Could you check a few things on this drawing? It's one solid part, dimensions in mm from its lowest x, y, z. A direction names the side the tool comes from. Round coordinates to 2 decimals unless told otherwise and drop trailing zeros. Loops run counter-clockwise (first coordinate to the right, second up) from the corner with the lowest first, then second, coordinate; pieces in that order, holes last. Notation, with made-up numbers: (53, -17.75) -> (64, -17.75) arc R27 ccw to (64, 21.25) -> close; hole circle Ø2 at (30.25, 8.5). An arc over 180 degrees is marked (long way). Use one line per item in the form item = value. Start each with the question number.
Item 1: If we section it at C-C (y = 3): Write out the boundary of the cut face in (x, z), then the cut area to 3 significant figures.
Item 2: I'm going to push flat-ended pins straight in: pin 1 Ø5 at (y, z) = (27.5, 10) entering from -X; pin 2 Ø1.4 at (x, y) = (31, 37) entering from -Z. Where does each tip first touch, or does it pass through?
Item 3: If I drill on L1, parallel to Y at x = 31, z = 1.8; L2, parallel to Z at x = 37.6, y = 11; L3, parallel to Z at x = 29, y = 23, over which ranges is the centre line in solid material (lowest first)? Write a range as [from, to].
Item 4: If we section it at B-B (x = 31): Write out the boundary of the cut face in (y, z), then the cut area to 3 significant figures.
Item 5: If we section it at D-D (y = 32): Write out the boundary of the cut face in (x, z).
Item 6: If we section it at A-A (z = 10): Write out the boundary of the cut face in (x, y), then the cut area to 3 significant figures.
Item 7: For the marked faces 1 and 2, which set-ups out of +Z, -Z, +X, -X, +Y, -Y let a thin tool reach every point of the face, with its end or its side?
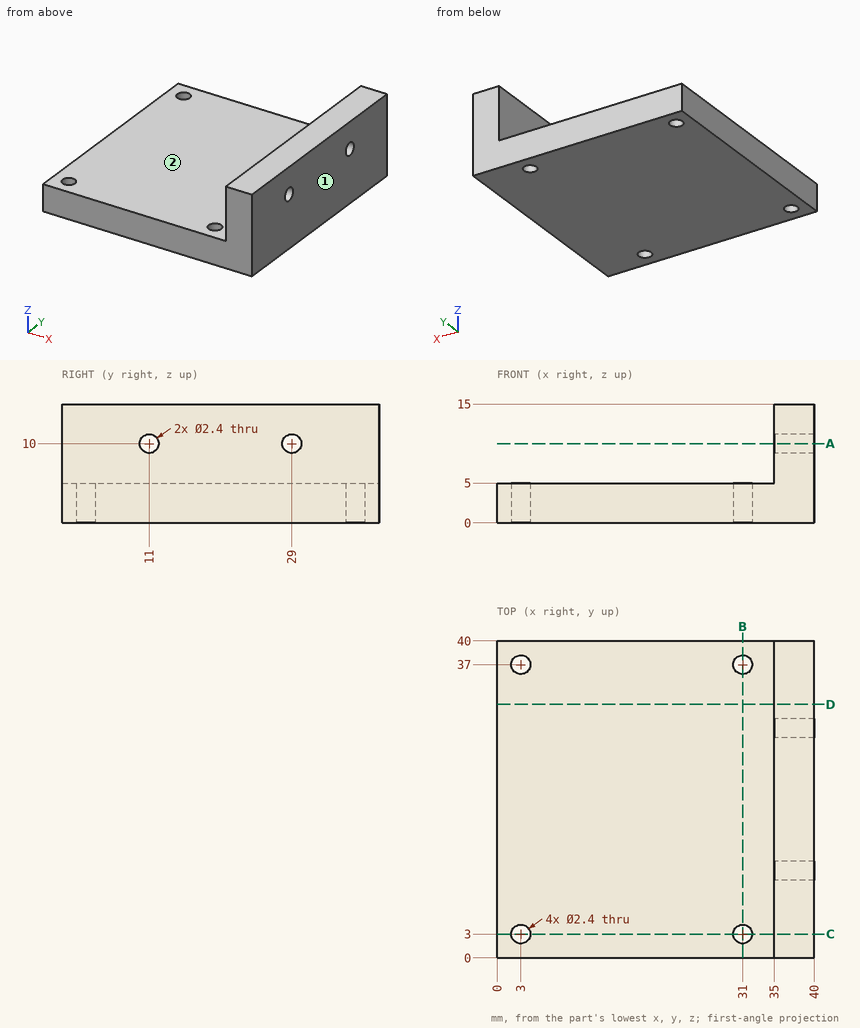
Values found:
q1.outline = (0, 0) -> (1.8, 0) -> (1.8, 5) -> (0, 5) -> close; (4.2, 0) -> (29.8, 0) -> (29.8, 5) -> (4.2, 5) -> close; (32.2, 0) -> (40, 0) -> (40, 15) -> (35, 15) -> (35, 5) -> (32.2, 5) -> close
q1.area = 226 mm2
q2.pin_1 = 35
q2.pin_2 = through
q3.L1 = [0, 1.8], [4.2, 35.8], [38.2, 40]
q3.L2 = [0, 8.8], [11.2, 15]
q3.L3 = [0, 5]
q4.outline = (0, 0) -> (1.8, 0) -> (1.8, 5) -> (0, 5) -> close; (4.2, 0) -> (35.8, 0) -> (35.8, 5) -> (4.2, 5) -> close; (38.2, 0) -> (40, 0) -> (40, 5) -> (38.2, 5) -> close
q4.area = 176 mm2
q5.outline = (0, 0) -> (40, 0) -> (40, 15) -> (35, 15) -> (35, 5) -> (0, 5) -> close
q6.outline = (35, 0) -> (40, 0) -> (40, 9.8) -> (35, 9.8) -> close; (35, 12.2) -> (40, 12.2) -> (40, 27.8) -> (35, 27.8) -> close; (35, 30.2) -> (40, 30.2) -> (40, 40) -> (35, 40) -> close
q6.area = 176 mm2
q7.face_1 = +Z, -Z, +X, +Y, -Y
q7.face_2 = +Z, -X, +Y, -Y
